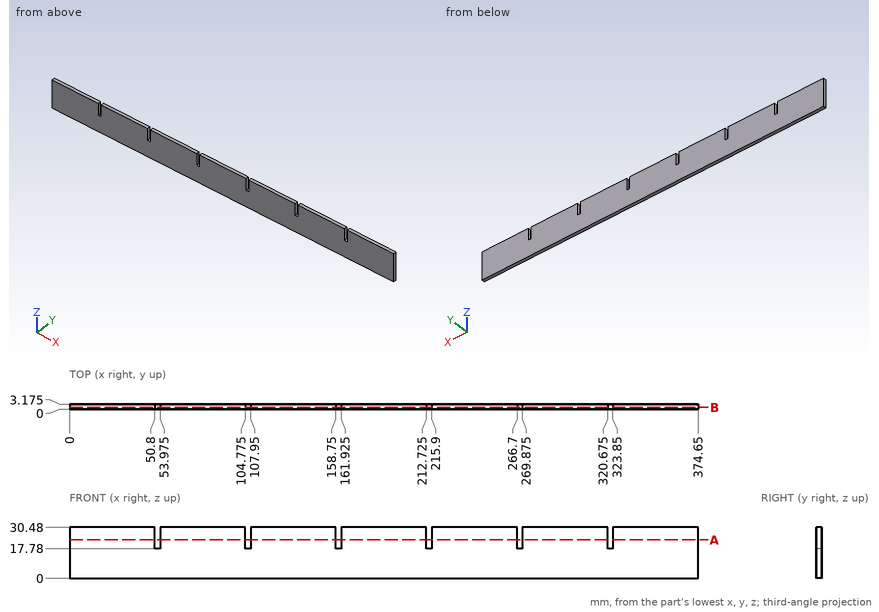
Design review of the part shown in the three views and the two pictorial views. Dimensions are in mm from the part's minimum x, y and z. Round coordinates to 2 decimals unless told otherwise and drop trailing zeros. Order: outer loops, then holes, each group sorted by start corner. A loop starts at its lowest first (then second) coordinate and runs counter-clockwise, first axis right, second up.
Item 1: To check wall thickness, follow probe 1 along Z at (x, y) = (53, 2.2). State the ranges of the line that lie inside material, in increasing order.
Working result:
probe 1: z = 0 to 17.78
Item 2: Add section A-A, the plane z = 23. State the section outline as (x, y) points (3 decimals).
Working result:
outline: (0, 0) - (50.8, 0) - (50.8, 3.175) - (0, 3.175) - close; (53.975, 0) - (104.775, 0) - (104.775, 3.175) - (53.975, 3.175) - close; (107.95, 0) - (158.75, 0) - (158.75, 3.175) - (107.95, 3.175) - close; (161.925, 0) - (212.725, 0) - (212.725, 3.175) - (161.925, 3.175) - close; (215.9, 0) - (266.7, 0) - (266.7, 3.175) - (215.9, 3.175) - close; (269.875, 0) - (320.675, 0) - (320.675, 3.175) - (269.875, 3.175) - close; (323.85, 0) - (374.65, 0) - (374.65, 3.175) - (323.85, 3.175) - close
Item 3: For pin 1 (1.6 mm diameter, centred on x = 322.5, y = 2, fed in from +Z), flat-tipped, find the tip position at first contact; note if it passes through.
Working result:
pin 1: stops at z = 17.78
Item 4: Add section B-B, the plane y = 1.1. State the section outline as (x, z) points (3 decimals), and give its area (3 significant figures).
Working result:
outline: (0, 0) - (374.65, 0) - (374.65, 30.48) - (323.85, 30.48) - (323.85, 17.78) - (320.675, 17.78) - (320.675, 30.48) - (269.875, 30.48) - (269.875, 17.78) - (266.7, 17.78) - (266.7, 30.48) - (215.9, 30.48) - (215.9, 17.78) - (212.725, 17.78) - (212.725, 30.48) - (161.925, 30.48) - (161.925, 17.78) - (158.75, 17.78) - (158.75, 30.48) - (107.95, 30.48) - (107.95, 17.78) - (104.775, 17.78) - (104.775, 30.48) - (53.975, 30.48) - (53.975, 17.78) - (50.8, 17.78) - (50.8, 30.48) - (0, 30.48) - close
area: 11,200 mm2
